For this review, take the finished solid that the model builds, in its own axes (mm). A direction names the side the tool comes from. Round coordinates to 2 decimals unless told otherwise and drop trailing zeros. Write each loop counter-clockwise with the first axis right and the second up, starting at its lowest first coordinate (ties: lowest second). Pieces come first, ordered by that corner, then holes.
from build123d import *

# Parameters (mm, degrees)
SKETCH1_W           = 41
SKETCH1_H           = 70
SKETCH1_R           = 3.3
BOSS_EXTRUDE1_DEPTH = 8
SKETCH2_R           = 5.5
CUT_EXTRUDE1_DEPTH  = 4.2
CHAMFER2_SIZE       = 3.2
FILLET1_R           = 4
CHAMFER4_SIZE       = 0.5


with BuildPart() as part:
    # Sketch1 → Boss-Extrude1 (new body)
    with BuildSketch(Plane(origin=(0, 0, 0), x_dir=(1, 0, 0), z_dir=(0, 1, 0))):
        Rectangle(SKETCH1_W, SKETCH1_H)
        with Locations((0, 17.5)):
            Circle(SKETCH1_R, mode=Mode.SUBTRACT)
        with Locations((0, -17.5)):
            Circle(SKETCH1_R, mode=Mode.SUBTRACT)
    extrude(amount=BOSS_EXTRUDE1_DEPTH)

    # Sketch2 → Cut-Extrude1 (cut)
    with BuildSketch(Plane(origin=(0, 8, 0), x_dir=(1, 0, 0), z_dir=(0, 1, 0))):
        with Locations((0, -17.5)):
            Circle(SKETCH2_R)
    extrude(amount=-CUT_EXTRUDE1_DEPTH, mode=Mode.SUBTRACT)

    # Chamfer2
    chamfer2_edges = [part.edges().sort_by_distance(p)[0] for p in [
        (-3.3, 8, -17.5),
    ]]
    chamfer(chamfer2_edges, length=CHAMFER2_SIZE)

    # Fillet1
    fillet1_edges = [part.edges().sort_by_distance(p)[0] for p in [
        (20.5, 4, 35),
        (-20.5, 4, 35),
        (-20.5, 4, -35),
        (20.5, 4, -35),
    ]]
    fillet(fillet1_edges, radius=FILLET1_R)

    # Chamfer4
    chamfer4_edges = [part.edges().sort_by_distance(p)[0] for p in [
        (0, 0, 35),
        (0, 8, 35),
        (20.5, 0, 0),
        (-20.5, 0, 0),
        (0, 0, -35),
        (-19.328427125, 0, -33.828427125),
        (19.328427125, 0, -33.828427125),
        (19.328427125, 0, 33.828427125),
        (-19.328427125, 0, 33.828427125),
        (-20.5, 8, 0),
        (20.5, 8, 0),
        (0, 8, -35),
        (-19.328427125, 8, -33.828427125),
        (19.328427125, 8, -33.828427125),
        (19.328427125, 8, 33.828427125),
        (-19.328427125, 8, 33.828427125),
    ]]
    chamfer(chamfer4_edges, length=CHAMFER4_SIZE)


solid = part.part
(1) For line 1 along Z through (x, y) = (0, 3); line 2 along X through (y, z) = (2.3, 17.5); line 3 along Z through (x, y) = (4.5, 7), list the stretches that pass through material, from the lowest coordinate up.
Geometry check:
line 1: z = -35 to -20.8, -14.2 to 14.2, 20.8 to 35
line 2: x = -20.5 to -3.3, 3.3 to 20.5
line 3: z = -35 to -20.66, -14.34 to 14.34, 20.66 to 35
(2) For pin 1 Ø3.5 at (x, z) = (0, 19.5) entering from +Y, flat-tipped, find the tip position at first contact; note if it passes through.
Geometry check:
pin 1: stops at y = 3.8
(3) We need section D-D, the plane z = 17.5. Give the boundary of the cut face in (x, y).
Geometry check:
outline: (-20.5, 0.5) - (-20, 0) - (-3.3, 0) - (-3.3, 3.8) - (-5.5, 3.8) - (-5.5, 8) - (-20, 8) - (-20.5, 7.5) - close; (3.3, 0) - (20, 0) - (20.5, 0.5) - (20.5, 7.5) - (20, 8) - (5.5, 8) - (5.5, 3.8) - (3.3, 3.8) - close
(4) For faces 1 (the face through (0, 3.8, 21)), 2 (the face through (-0.43, 1.87, 14.23)), list the 3-axis set-ups (+Z, -Z, +X, -X, +Y, -Y) from which the entire face can be reached by the end or side of a thin tool; tool diameter is ignored.
Geometry check:
face 1: +Y
face 2: +Y, -Y
(5) We need section B-B, the plane x = 0. Give the boundary of the cut face in (y, z).
Geometry check:
outline: (0, -34.5) - (0.5, -35) - (7.5, -35) - (8, -34.5) - (8, -24) - (4.8, -20.8) - (0, -20.8) - close; (0, -14.2) - (4.8, -14.2) - (8, -11) - (8, 12) - (3.8, 12) - (3.8, 14.2) - (0, 14.2) - close; (0, 20.8) - (3.8, 20.8) - (3.8, 23) - (8, 23) - (8, 34.5) - (7.5, 35) - (0.5, 35) - (0, 34.5) - close
(6) We need section C-C, the plane y = 6. Give the boundary of the cut face in (x, z), and give its area (3 significant figures).
Geometry check:
outline: (-20.5, -31) arc R4 ccw to (-16.5, -35) - (16.5, -35) arc R4 ccw to (20.5, -31) - (20.5, 31) arc R4 ccw to (16.5, 35) - (-16.5, 35) arc R4 ccw to (-20.5, 31) - close; hole circle Ø11 at (0, 17.5); hole circle Ø9 at (0, -17.5)
area: 2,700 mm2
(7) Mouldability with a two-part tool opening along Z and no side actions: class faces 3 (the face through (-19.1, 7.86, 33.55)), 4 (the face through (0, 4, -35)), 5 (the face through (-0.72, 2.37, -14.28)) as pulls with the +Z half, pulls with the -Z half, needs draft (parallel to the pull), parting line crosses it, or undercut.
Geometry check:
face 3: pulls with the +Z half
face 4: pulls with the -Z half
face 5: undercut
(8) We need section A-A, the plane z = -17.5. Give the boundary of the cut face in (x, y), and give its area (3 significant figures).
Geometry check:
outline: (-20.5, 0.5) - (-20, 0) - (-3.3, 0) - (-3.3, 4.8) - (-6.5, 8) - (-20, 8) - (-20.5, 7.5) - close; (3.3, 0) - (20, 0) - (20.5, 0.5) - (20.5, 7.5) - (20, 8) - (6.5, 8) - (3.3, 4.8) - close
area: 264 mm2
